```python
from build123d import *

# Parameters (mm, degrees)
SKETCH_1_W          = 164
SKETCH_1_H          = 180
EXTRUDE_1_DEPTH     = 10
SKETCH_2_W          = 4.88
SKETCH_2_H          = 159.88
EXTRUDE_2_DEPTH     = 10
SKETCH_3_R          = 2
CUT_EXTRUDE_1_DEPTH = 10
SKETCH_5_R          = 2.5
SKETCH_5_W          = 37
SKETCH_5_H          = 55
CUT_EXTRUDE_3_DEPTH = 8
SKETCH_6_W          = 37
SKETCH_6_H          = 55
CUT_EXTRUDE_4_DEPTH = 8


with BuildPart() as part:
    # 草图1 → 凸台-拉伸1 (new body)
    with BuildSketch(Plane.XY):
        with Locations((82, 90)):
            Rectangle(SKETCH_1_W, SKETCH_1_H)
    extrude(amount=EXTRUDE_1_DEPTH)

    # 草图2 → 凸台-拉伸2 (add)
    with BuildSketch(Plane.ZY):
        with Locations((5, 90)):
            Rectangle(SKETCH_2_W, SKETCH_2_H)
    extrude_2 = extrude(amount=EXTRUDE_2_DEPTH)

    # 镜向1: 凸台-拉伸2 across plane
    add(extrude_2.mirror(Plane(origin=(82, 0, 0), x_dir=(0, 0, 1), z_dir=(1, 0, 0))))

    # 草图3 → 切除-拉伸1 (cut)
    with BuildSketch(Plane(origin=(0, 0, 0), x_dir=(-1, 0, 0), z_dir=(0, 0, -1))):
        with Locations((-150.6425573, 145)):
            Circle(SKETCH_3_R)
        with Locations((-131.5, 157.75)):
            Circle(SKETCH_3_R)
        with Locations((-131.5, 132.25)):
            Circle(SKETCH_3_R)
        with Locations((-13.3574427, 145)):
            Circle(SKETCH_3_R)
        with Locations((-32.5, 157.75)):
            Circle(SKETCH_3_R)
        with Locations((-32.5, 132.25)):
            Circle(SKETCH_3_R)
        with Locations(Location((-131.5, 47.75, 0), (0, 0, 180))):
            Circle(SKETCH_3_R)
        with Locations(Location((-131.5, 22.25, 0), (0, 0, 180))):
            Circle(SKETCH_3_R)
        with Locations(Location((-150.6425573, 35, 0), (0, 0, 180))):
            Circle(SKETCH_3_R)
        with Locations(Location((-32.5, 47.75, 0), (0, 0, 180))):
            Circle(SKETCH_3_R)
        with Locations(Location((-32.5, 22.25, 0), (0, 0, 180))):
            Circle(SKETCH_3_R)
        with Locations(Location((-13.3574427, 35, 0), (0, 0, 180))):
            Circle(SKETCH_3_R)
    extrude(amount=-CUT_EXTRUDE_1_DEPTH, mode=Mode.SUBTRACT)

    # 草图5 → 切除-拉伸3 (cut)
    with BuildSketch(Plane.XY.offset(10)):
        with Locations((85.117863175, 105)):
            Circle(SKETCH_5_R)
        with Locations((85.117863175, 75)):
            Circle(SKETCH_5_R)
        with Locations((105.117863175, 105)):
            Circle(SKETCH_5_R)
        with Locations((105.117863175, 75)):
            Circle(SKETCH_5_R)
        with Locations((137.617863175, 90)):
            Rectangle(SKETCH_5_W, SKETCH_5_H)
    extrude(amount=-CUT_EXTRUDE_3_DEPTH, mode=Mode.SUBTRACT)

    # 草图6 → 切除-拉伸4 (cut)
    with BuildSketch(Plane.XY.offset(2)):
        with Locations((137.617863175, 90)):
            Rectangle(SKETCH_6_W, SKETCH_6_H)
    extrude(amount=-CUT_EXTRUDE_4_DEPTH, mode=Mode.SUBTRACT)


solid = part.part
```
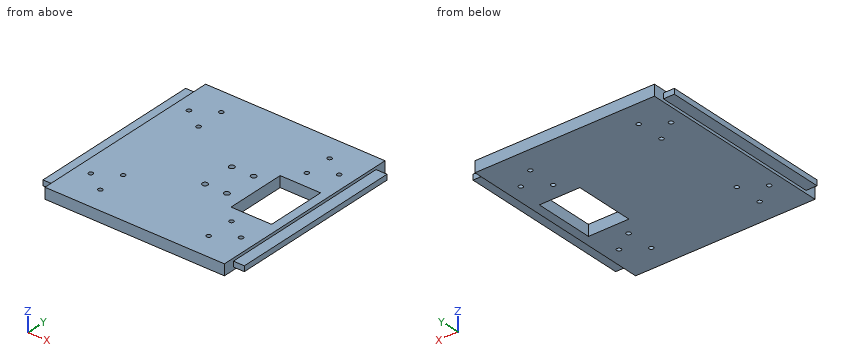
CAD build for the part. Positions are in the model's coordinates, mm. Coordinates: 2 decimals unless noted, no trailing zeros. Write each loop counter-clockwise with the first axis right and the second up, starting at its lowest first coordinate (ties: lowest second). Pieces come first, ordered by that corner, then holes. Notation, with made-up numbers: (-26, 47.25) -> (6, 47.25) arc R21 ccw to (6, 76.25) -> close; hole circle Ø8 at (70.5, -9.5). An arc over 180 degrees is marked (long way). Use CSV: the item, a comma, the result in double quotes. Start each with the question number.
Item 1: Band-saw the part on A-A, the plane y = 100. Write the cut outline in (x, z), plus the area to 3 significant figures.
Item 2: Band-saw the part on D-D, the plane y = 59.5. Write the cut outline in (x, z).
Item 3: Band-saw the part on B-B, the plane x = 124.5. Write the cut outline in (y, z).
Item 4: Drop flat-ended pins along their axis: P1, Ø3, axis at x = 171, y = 105, coming from the +Z side; P2, Ø3, axis at x = -4, y = 92.5, coming from the -Z side; P3, Ø3.5, axis at x = 32.5, y = 22.25, coming from the -Z side; P4, Ø2.5, axis at x = 105, y = 105.5, coming from the +Z side. Give the stop position or say it passes through.
Item 5: Wall check: probe 1 along Y at (x, z) = (32.5, 6.75); probe 2 along X at (y, z) = (145, 6.25); probe 3 along Y at (x, z) = (146, 6.75). Give the ranges that are in metal, low to high.
Item 6: Band-saw the part on C-C, the plane z = 5. Give the number of separate pieces and of enclosed holes in the cut face, plus the area to 3 significant figures.
Response values:
1,outline,"(-10, 2.56) -> (0, 2.56) -> (0, 0) -> (119.12, 0) -> (119.12, 10) -> (0, 10) -> (0, 7.44) -> (-10, 7.44) -> close; (156.12, 0) -> (164, 0) -> (164, 2.56) -> (174, 2.56) -> (174, 7.44) -> (164, 7.44) -> (164, 10) -> (156.12, 10) -> close"
1,area,"1,370 mm2"
2,outline,"(-10, 2.56) -> (0, 2.56) -> (0, 0) -> (164, 0) -> (164, 2.56) -> (174, 2.56) -> (174, 7.44) -> (164, 7.44) -> (164, 10) -> (0, 10) -> (0, 7.44) -> (-10, 7.44) -> close"
3,outline,"(0, 0) -> (62.5, 0) -> (62.5, 10) -> (0, 10) -> close; (117.5, 0) -> (180, 0) -> (180, 10) -> (117.5, 10) -> close"
4,P1,"stops at z = 7.44"
4,P2,"stops at z = 2.56"
4,P3,"passes through"
4,P4,"stops at z = 2"
5,probe 1,"y = 0 to 20.25, 24.25 to 45.75, 49.75 to 130.25, 134.25 to 155.75, 159.75 to 180"
5,probe 2,"x = -10 to 11.36, 15.36 to 148.64, 152.64 to 174"
5,probe 3,"y = 0 to 62.5, 117.5 to 180"
6,separate pieces,"1"
6,enclosed holes,"17"
6,area,"30,500 mm2"
